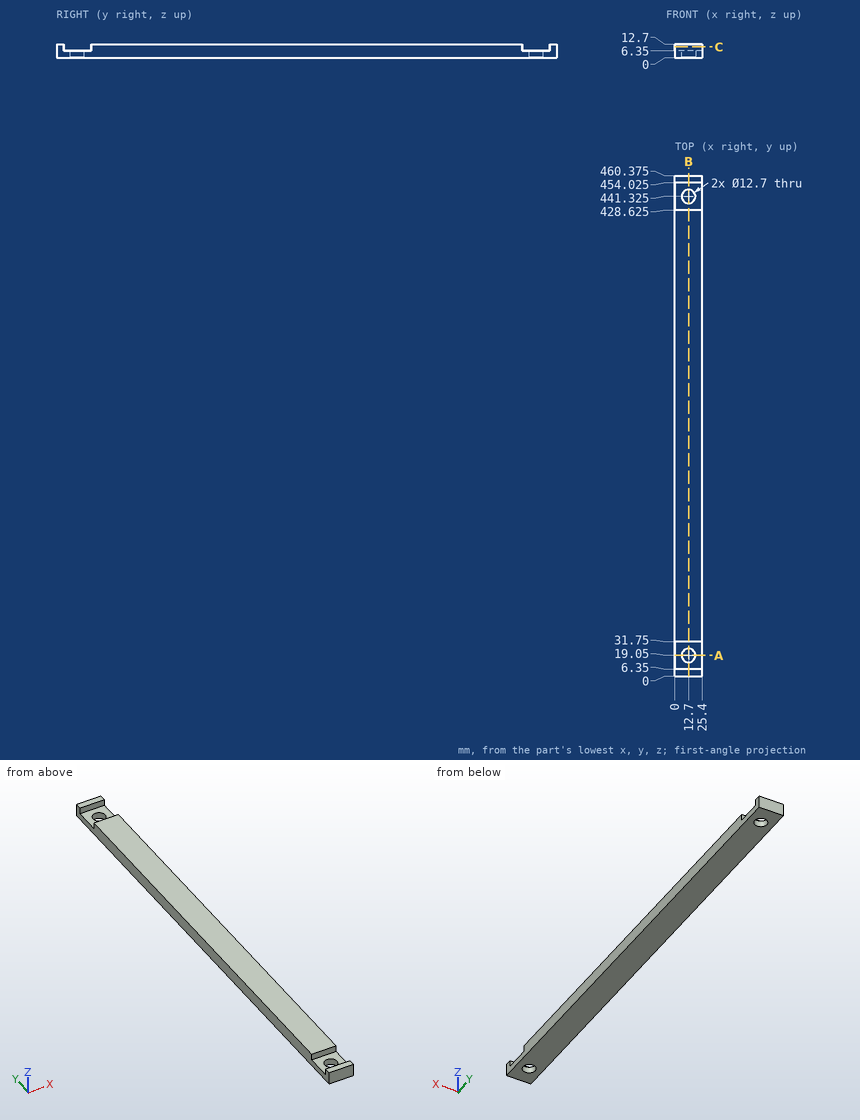
The figure shows three views and two pictorial views of one solid part (mm, origin at its lowest corner). Answer the questions. Coordinates: 2 decimals unless noted, no trailing zeros. Loops run counter-clockwise (first coordinate to the right, second up) from the corner with the lowest first, then second, coordinate; pieces in that order, holes last. Notation, with made-up numbers: (71.25, 29.5) -> (106.25, 29.5) arc R24 ccw to (106.25, 57.5) -> close; hole circle Ø9 at (16.5, -7). An arc over 180 degrees is marked (long way). Use one line per item in the form item = value. Start each with the question number.
Item 1: The part is cut by section C-C on z = 10. Determine the outline of the cut face in (x, y) (3 decimals), then the cut area to 3 significant figures.
Item 2: Consider L1, parallel to Y at x = 12.7, z = 3 (3 decimals); L2, parallel to Y at x = 11, z = 11.5 (3 decimals). Determine where each line is inside the solid, lowest interval first. Write a range as [from, to].
Item 3: The part is cut by section B-B on x = 12.7. Determine the outline of the cut face in (y, z) (3 decimals), then the cut area to 3 significant figures.
Item 4: The part is cut by section A-A on y = 19.05. Determine the outline of the cut face in (x, z), then the cut area to 3 significant figures.
Item 5: Flat-ended cylindrical pins translate along their axes: pin 1 Ø12.5 at (x, y) = (12, 441.5) entering from +Z; pin 2 Ø4 at (x, z) = (18.5, 6.5) entering from -Y. Find the tip coordinate at first contact, or state that the pin passes through.
Answer key:
q1.outline = (0, 0) -> (25.4, 0) -> (25.4, 6.35) -> (0, 6.35) -> close; (0, 31.75) -> (25.4, 31.75) -> (25.4, 428.625) -> (0, 428.625) -> close; (0, 454.025) -> (25.4, 454.025) -> (25.4, 460.375) -> (0, 460.375) -> close
q1.area = 10,400 mm2
q2.L1 = [0, 12.7], [25.4, 434.975], [447.675, 460.375]
q2.L2 = [0, 6.35], [31.75, 428.625], [454.025, 460.375]
q3.outline = (0, 0) -> (12.7, 0) -> (12.7, 6.35) -> (6.35, 6.35) -> (6.35, 12.7) -> (0, 12.7) -> close; (25.4, 0) -> (434.975, 0) -> (434.975, 6.35) -> (428.625, 6.35) -> (428.625, 12.7) -> (31.75, 12.7) -> (31.75, 6.35) -> (25.4, 6.35) -> close; (447.675, 0) -> (460.375, 0) -> (460.375, 12.7) -> (454.025, 12.7) -> (454.025, 6.35) -> (447.675, 6.35) -> close
q3.area = 5,360 mm2
q4.outline = (0, 0) -> (6.35, 0) -> (6.35, 6.35) -> (0, 6.35) -> close; (19.05, 0) -> (25.4, 0) -> (25.4, 6.35) -> (19.05, 6.35) -> close
q4.area = 80.6 mm2
q5.pin_1 = 6.35
q5.pin_2 = 0
